from build123d import *

# Parameters (mm, degrees)
BOSS_EXTRUDE1_DEPTH                = 25.4
F_25_64_0_39063_DIAMETER_HOLE1_D   = 9.922002
CIRPATTERN4_COUNT                  = 36
TAPPED_HOLE_FOR_1_2_13_HELICOIL1_D = 13.09624
LPATTERN1_COUNT                    = 4
LPATTERN1_PITCH                    = 69.85


with BuildPart() as part:
    # Sketch1 → Boss-Extrude1 (new body)
    with BuildSketch(Plane(origin=(0, 0, 0), x_dir=(1, 0, 0), z_dir=(0, 1, 0))):
        with BuildLine():
            Line((-152.4, 677.116373325), (-152.4, 717.55))
            Line((-152.4, 717.55), (152.4, 717.55))
            Line((152.4, 717.55), (152.4, 677.116373325))
            ThreePointArc((152.4, 677.116373325), (0, 694.055), (-152.4, 677.116373325))
        make_face()
    extrude(amount=BOSS_EXTRUDE1_DEPTH)

    # 25/64 (0.39063) Diameter Hole1 (through all)
    with Locations(Plane(origin=(0, 25.4, 0), x_dir=(1, 0, 0), z_dir=(0, 1, 0))):
        with Locations((0, 702.5)):
            f_25_64_0_39063_diameter_hole1 = Hole(F_25_64_0_39063_DIAMETER_HOLE1_D / 2)

    # CirPattern4: 25/64 (0.39063) Diameter Hole1 ×36 about axis, 33 skipped
    cirpattern4_axis = Axis((0, 0, 0), (0, -1, 0))
    add([f_25_64_0_39063_diameter_hole1.rotate(cirpattern4_axis, i * 360 / CIRPATTERN4_COUNT) for i in range(1, CIRPATTERN4_COUNT) if i not in (2, 3, 4, 5, 6, 7, 8, 9, 10, 11, 12, 13, 14, 15, 16, 17, 18, 19, 20, 21, 22, 23, 24, 25, 26, 27, 28, 29, 30, 31, 32, 33, 34)], mode=Mode.SUBTRACT)

    # Tapped Hole for 1/2-13 Helicoil1 (through all)
    with Locations(Plane(origin=(0, 0, -717.55), x_dir=(-1, 0, 0), z_dir=(0, 0, -1))):
        with Locations((-104.775, 12.7)):
            tapped_hole_for_1_2_13_helicoil1 = Hole(TAPPED_HOLE_FOR_1_2_13_HELICOIL1_D / 2)

    # LPattern1: Tapped Hole for 1/2-13 Helicoil1 ×4
    with Locations(*[(-i * LPATTERN1_PITCH, 0, 0) for i in range(1, LPATTERN1_COUNT)]):
        add(tapped_hole_for_1_2_13_helicoil1, mode=Mode.SUBTRACT)


solid = part.part
Design review of the part built by this model. Coordinates are the model's own, in mm. Give positions to 0.01 mm unless a question says otherwise; leave off trailing zeros. Loops run counter-clockwise (first coordinate to the right, second up) from the corner with the lowest first, then second, coordinate; pieces in that order, holes last. Notation, with made-up numbers: M 37.25,28.25 L 91.25,28.25 A21 ccw 91.25,36.25 Z; hole C 65,55 d2. An arc over 180 degrees is marked long. Answer as a JSON object with one key per item and string values.
Item 1: We need section C-C (y = 12.7). State the section outline as (x, z) points (3 decimals).
Output values:
{"outline": "M -152.4,-717.55 L -111.323,-717.55 L -111.323,-685.069 A694.055 cw -152.4,-677.116 Z; M -98.227,-717.55 L -41.473,-717.55 L -41.473,-692.815 A694.055 cw -98.227,-687.069 Z; M -28.377,-717.55 L 28.377,-717.55 L 28.377,-693.475 A694.055 cw -28.377,-693.475 Z; M 41.473,-717.55 L 98.227,-717.55 L 98.227,-687.069 A694.055 cw 41.473,-692.815 Z; M 111.323,-717.55 L 152.4,-717.55 L 152.4,-677.116 A694.055 cw 111.323,-685.069 Z; hole C -121.988,-691.827 d9.922; hole C 0,-702.5 d9.922; hole C 121.988,-691.827 d9.922"}
Item 2: Wall thickness on line 1 along X through (y, z) = (12.7, -707.5); line 2 along X through (y, z) = (12.7, -703); line 3 along X through (y, z) = (20, -702.5): over which ranges is each line inside the solid? List them lowest first.
Output values:
{"line 1": "x = -152.4 to -111.32, -98.23 to -41.47, -28.38 to 28.38, 41.47 to 98.23, 111.32 to 152.4", "line 2": "x = -152.4 to -111.32, -98.23 to -41.47, -28.38 to -4.94, 4.94 to 28.38, 41.47 to 98.23, 111.32 to 152.4", "line 3": "x = -152.4 to -4.96, 4.96 to 152.4"}
Item 3: Mouldability with a two-part tool opening along Y and no side actions: class faces 1 (the face through (-111.317, 12.988, -701.082)), 2 (the face through (152.4, 13, -698)), 3 (the face through (2.1, 0, -697.6)) as pulls with the +Y half, pulls with the -Y half, needs draft (parallel to the pull), parting line crosses it, or undercut.
Output values:
{"face 1": "undercut", "face 2": "needs draft", "face 3": "pulls with the -Y half"}
Item 4: We need section A-A (z = -702.5). State the section outline as (x, y) points (3 decimals), and give its area (3 significant figures).
Output values:
{"outline": "M -152.4,0 L -4.961,0 L -4.961,25.4 L -152.4,25.4 Z; M 4.961,0 L 152.4,0 L 152.4,25.4 L 4.961,25.4 Z; hole C -104.775,12.7 d13.096; hole C -34.925,12.7 d13.096; hole C 34.925,12.7 d13.096; hole C 104.775,12.7 d13.096", "area": "6,950 mm2"}
Item 5: We need section D-D (z = -714). State the section outline as (x, y) points (3 decimals), and give its area (3 significant figures).
Output values:
{"outline": "M -152.4,0 L 152.4,0 L 152.4,25.4 L -152.4,25.4 Z; hole C -104.775,12.7 d13.096; hole C -34.925,12.7 d13.096; hole C 34.925,12.7 d13.096; hole C 104.775,12.7 d13.096", "area": "7,200 mm2"}
Item 6: We need section B-B (x = 0). State the section outline as (y, z) points (3 decimals), and give its area (3 significant figures).
Output values:
{"outline": "M 0,-717.55 L 25.4,-717.55 L 25.4,-707.461 L 0,-707.461 Z; M 0,-697.539 L 25.4,-697.539 L 25.4,-694.055 L 0,-694.055 Z", "area": "345 mm2"}
Item 7: For P1, Ø5, axis at x = -71.5, y = 11.5, coming from the +Z side, flat-tipped, find the tip position at first contact; note if it passes through.
Output values:
{"P1": "stops at z = -690.1"}
